Solid Edge part; units mm, degrees
sketch "Sketch1" plane through (0, 0, 0) normal (0, 0, 1) x (1, 0, 0)
  line L0 (-0.7217, 1.25) -> (0.7217, 1.25)
  line L1 (0.7217, 1.25) -> (1.4434, 0)
  line L2 (1.4434, 0) -> (0.7217, -1.25)
  line L3 (0.7217, -1.25) -> (-0.7217, -1.25)
  line L4 (-0.7217, -1.25) -> (-1.4434, 0)
  line L5 (-1.4434, 0) -> (-0.7217, 1.25)
  circle A0 centre (0, 0) radius 2.75
extrude "Protrusion1" add sketch "Sketch1" along normal blind 3
sketch "Sketch2" plane through (0, 0, 0) normal (0, -1, 0) x (1, 0, 0)
  line L0 (0, 0.8667) -> (1.4434, 1.7)
  line L1 (1.4434, 1.7) -> (2.75, 1.7)
  line L2 (2.75, 1.7) -> (2.75, 0)
  line L3 (2.75, 0) -> (1.5, 0)
  line L4 (1.5, 0) -> (1.5, -21.999)
  line L5 (1.5, -21.999) -> (1.5, -22) construction
  line L6 (1.5, -22) -> (1.5, -22) construction
  line L7 (1.5, -22) -> (1.5, -40)
  line L8 (0, -40) -> (1.5, -40)
revolve "RevolvedProtrusion_1" add sketch "Sketch2" angle 360 about axis through (0, 0, 2.3333) along (0, 0, -1)
cosmetic_thread "Thread_1" thread depth 17.999
sketch "Sketch3" plane through (0, 0, 0) normal (0, -1, 0) x (1, 0, 0)
  line L0 (0, 4) -> (1.435, 4)
  line L1 (1.435, 4) -> (1.435, 3)
  line L2 (1.435, 3) -> (0, 2.1715)
revolve "RevolvedCutout_1" cut sketch "Sketch3" angle 360 about axis through (0, 0, 7.1999) along (0, 0, 1)
fillet "Round_1" radius 0.3 1 edges at (-2.75, 0, 3)
sketch "Sketch4" plane through (0, 0, 0) normal (0, -1, 0) x (1, 0, 0)
  line L0 (1.5, 0) -> (1.8, 0)
  arc A0 (1.7101, -0.0562) -> (1.8, 0) centre (1.8, -0.1) cw
  line L1 (1.5101, -0.4662) -> (1.7101, -0.0562)
  arc A1 (1.5101, -0.4662) -> (1.5, -0.51) centre (1.6, -0.51) ccw
  line L2 (1.5, 0) -> (1.5, -0.51)
revolve "RevolvedProtrusion_2" add sketch "Sketch4" angle 360 about axis through (0, 0, -1.02) along (0, 0, 1)
chamfer "Chamfer_1" distance 0.2705 angle 45 1 edges at (-1.5, 0, -40)
properties material "Steel"
The listing builds one solid part. Answer for the finished solid, in the listing's coordinates (mm). A direction names the side the tool comes from. Coordinates: 2 decimals unless noted, no trailing zeros. Loops run counter-clockwise (first coordinate to the right, second up) from the corner with the lowest first, then second, coordinate; pieces in that order, holes last. Notation, with made-up numbers: (35, -17.75) -> (53, -17.75) arc R33 cw to (53, 13.25) -> close; hole circle Ø11 at (22, 57). An arc over 180 degrees is marked (long way). Write item = value, one per line. Start each with the question number.
1) A tool of negligible diameter and unlimited length cuts with its end or side. For faces 4 (the face through (0, -2, 3)), 5 (the face through (1.08, 0.63, 2.28)), from which of +Z, -Z, +X, -X, +Y, -Y can it reach the whole face along a straight path? Write none if from no direction.
2) A cutting plane is placed at A-A (z = -11). Give the vertices of the cut face in (x, y), then the cut area to 3 significant figures.
3) Given pin 1 Ø2 at (y, z) = (0, -7) entering from +X, flat-ended and moving along its own axis, determine where the tip first touches the part or whether it passes through.
4) Straight lines are drawn through the part: line 1 (Z direction, x = -1.8, y = -1.05); line 2 (Z direction, x = 0.9, y = -0.65); line 3 (X direction, y = 0.25, z = 1.5). For each, find the intervals that lie inside material, in ascending order. Write a range as from..to.
5) The mould has two halves that part along X. Classify faces 1 (the face through (2, -1, 0)), 2 (the face through (-1.5, -0.07, -20.39)), 3 (the face through (1.088, -0.616, 2.284)): released by +X, released by -X, zero draft, split by the parting line, or undercut.
Responses:
q1.face_4 = +Z, +X, -X, +Y, -Y
q1.face_5 = +Z
q2.outline = circle Ø3 at (0, 0)
q2.area = 7.07 mm²
q3.pin_1 = 1.5
q4.line_1 = 0..3
q4.line_2 = -40..1.51
q4.line_3 = -2.74..-1.07, 1.07..2.74
q5.face_1 = zero draft
q5.face_2 = split by the parting line
q5.face_3 = undercut
